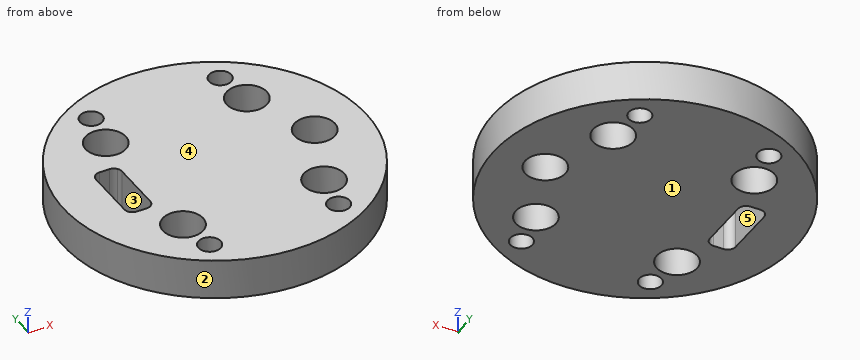
from build123d import *

# Parameters (mm, degrees)
SKETCH_1_R          = 37.5
EXTRUDE_1_DEPTH     = 10
SKETCH_2_R          = 5
CUT_EXTRUDE_1_DEPTH = 10
SKETCH_4_R          = 2.75
CUT_EXTRUDE_2_DEPTH = 10


with BuildPart() as part:
    # 草图1 → 凸台-拉伸1 (new body)
    with BuildSketch(Plane.XY):
        Circle(SKETCH_1_R)
        with BuildLine():
            ThreePointArc((-20.75113276, -17.528548354), (-17.528548354, -14.305963949), (-14.305963949, -17.528548354))
            ThreePointArc((-14.305963949, -17.528548354), (-17.528548354, -20.75113276), (-20.75113276, -17.528548354))
        make_face(mode=Mode.SUBTRACT)
        with BuildLine():
            ThreePointArc((14.305963949, -17.528548354), (17.528548354, -14.305963949), (20.75113276, -17.528548354))
            ThreePointArc((20.75113276, -17.528548354), (17.528548354, -20.75113276), (14.305963949, -17.528548354))
        make_face(mode=Mode.SUBTRACT)
        with BuildLine():
            Line((-24.045437487, 8.428297676), (-21.566526406, 8.428297676))
            ThreePointArc((-21.566526406, 8.428297676), (-20.68362959, 8.220920288), (-19.985383241, 7.642159365))
            ThreePointArc((-19.985383241, 7.642159365), (-19.686578169, 7.076512396), (-19.583397541, 6.445168811))
            Line((-19.583397541, 6.445168811), (-19.583397541, -6.445168811))
            ThreePointArc((-19.583397541, -6.445168811), (-20.164242538, -7.847452679), (-21.566526406, -8.428297676))
            Line((-21.566526406, -8.428297676), (-24.045437487, -8.428297676))
            ThreePointArc((-24.045437487, -8.428297676), (-25.447721356, -7.847452679), (-26.028566352, -6.445168811))
            Line((-26.028566352, -6.445168811), (-26.028566352, 6.445168811))
            ThreePointArc((-26.028566352, 6.445168811), (-25.447721356, 7.847452679), (-24.045437487, 8.428297676))
        make_face(mode=Mode.SUBTRACT)
        with BuildLine():
            ThreePointArc((-20.75113276, 17.528548354), (-17.528548354, 20.75113276), (-14.305963949, 17.528548354))
            ThreePointArc((-14.305963949, 17.528548354), (-17.528548354, 14.305963949), (-20.75113276, 17.528548354))
        make_face(mode=Mode.SUBTRACT)
        with BuildLine():
            ThreePointArc((14.305963949, 17.528548354), (17.528548354, 20.75113276), (20.75113276, 17.528548354))
            ThreePointArc((20.75113276, 17.528548354), (17.528548354, 14.305963949), (14.305963949, 17.528548354))
        make_face(mode=Mode.SUBTRACT)
        with BuildLine():
            ThreePointArc((21.814417514, 0), (24.789110812, 2.974693297), (27.763804109, 0))
            ThreePointArc((27.763804109, 0), (24.789110812, -2.974693297), (21.814417514, 0))
        make_face(mode=Mode.SUBTRACT)
    extrude(amount=EXTRUDE_1_DEPTH)

    # 草图2 → 切除-拉伸1 (cut)
    with BuildSketch(Plane.XY.offset(10)):
        with Locations((-17.528548354, 17.528548354)):
            Circle(SKETCH_2_R)
        with BuildLine():
            ThreePointArc((-20.75113276, 17.528548354), (-17.528548354, 14.305963949), (-14.305963949, 17.528548354))
            ThreePointArc((-14.305963949, 17.528548354), (-17.528548354, 20.75113276), (-20.75113276, 17.528548354))
        make_face(mode=Mode.SUBTRACT)
        with Locations((17.528548354, 17.528548354)):
            Circle(SKETCH_2_R)
        with BuildLine():
            ThreePointArc((20.75113276, 17.528548354), (17.528548354, 20.75113276), (14.305963949, 17.528548354))
            ThreePointArc((14.305963949, 17.528548354), (17.528548354, 14.305963949), (20.75113276, 17.528548354))
        make_face(mode=Mode.SUBTRACT)
        with Locations((-17.528548354, -17.528548354)):
            Circle(SKETCH_2_R)
        with BuildLine():
            ThreePointArc((-20.75113276, -17.528548354), (-17.528548354, -20.75113276), (-14.305963949, -17.528548354))
            ThreePointArc((-14.305963949, -17.528548354), (-17.528548354, -14.305963949), (-20.75113276, -17.528548354))
        make_face(mode=Mode.SUBTRACT)
        with Locations((17.528548354, -17.528548354)):
            Circle(SKETCH_2_R)
        with BuildLine():
            ThreePointArc((14.305963949, -17.528548354), (17.528548354, -20.75113276), (20.75113276, -17.528548354))
            ThreePointArc((20.75113276, -17.528548354), (17.528548354, -14.305963949), (14.305963949, -17.528548354))
        make_face(mode=Mode.SUBTRACT)
        with Locations((24.789110812, 0)):
            Circle(SKETCH_2_R)
        with BuildLine():
            ThreePointArc((21.814417514, 0), (24.789110812, -2.974693297), (27.763804109, 0))
            ThreePointArc((27.763804109, 0), (24.789110812, 2.974693297), (21.814417514, 0))
        make_face(mode=Mode.SUBTRACT)
    extrude(amount=-CUT_EXTRUDE_1_DEPTH, mode=Mode.SUBTRACT)

    # 草图4 → 切除-拉伸2 (cut)
    with BuildSketch(Plane.XY.offset(10)):
        with Locations((-16.071064876, -26.957760919)):
            Circle(SKETCH_4_R)
        with Locations((15.928824109, -27.042051743)):
            Circle(SKETCH_4_R)
        with Locations((16.071064876, 26.957760919)):
            Circle(SKETCH_4_R)
        with Locations((-15.928824109, 27.042051743)):
            Circle(SKETCH_4_R)
    extrude(amount=-CUT_EXTRUDE_2_DEPTH, mode=Mode.SUBTRACT)


solid = part.part
Design review of the part built by this model. Coordinates are the model's own, in mm. Face numbers are marked on the shaded views. A direction names the side the tool comes from. Round coordinates to 2 decimals unless told otherwise and drop trailing zeros. Write each loop counter-clockwise with the first axis right and the second up, starting at its lowest first coordinate (ties: lowest second). Pieces come first, ordered by that corner, then holes. Notation, with made-up numbers: (-24.75, -10.75) -> (-15.75, -10.75) arc R34 ccw to (-15.75, 23.25) -> close; hole circle Ø3 at (53, 80.5). An arc over 180 degrees is marked (long way). One line per item, written item: value. Start each with the question number.
Q1. To check wall thickness, follow probe 1 along X at (y, z) = (-16, 2); probe 2 along X at (y, z) = (-4, 4.5); probe 3 along Y at (x, z) = (15, 3.25). State the ranges of each line that lie inside material, in increasing order.
Q2. Add section C-C (z = 7.5). State how many separate pieces and enclosed holes the cut face has, then the cut area to 3 significant figures.
Q3. Add section D-D (y = -28). Give the boundary of the cut face in (x, z), then the cut area to 3 significant figures.
Q4. Tool access review of the marked faces 4 and 5: name each direction out of +Z, -Z, +X, -X, +Y, -Y from which nothing blocks a thin tool from reaching the whole face with its end or side.
Q5. Add section B-B (x = 28). Give the boundary of the cut face in (y, z).
Q6. Add section A-A (y = 0). Give the boundary of the cut face in (x, z), then the cut area to 3 significant figures.
Q7. The part is to be moulded in two halves that separate along Y. For the marked faces 1, 2 and 3, say which applies: pulls with the +Y half, pulls with the -Y half, needs draft (parallel to the pull), parting line crosses it, or undercut.
Q8. Insertion check: P1, Ø13, axis at x = 24.79, y = 0, coming from the -Z side; P2, Ø4, axis at y = 3, z = 3, coming from the -X side; P3, Ø0.7, axis at x = -22.5, z = 7.5, coming from the +Y side; P4, Ø4, axis at y = 22, z = 4, coming from the -X side. Each pin has a flat end and moves straight along its axis. Give the tip position at first contact, or say it passes through.
Response:
1. probe 1: x = -33.92 to -22.29, -12.77 to 12.77, 22.29 to 33.92
1. probe 2: x = -37.29 to -26.03, -19.58 to 21.79, 27.79 to 37.29
1. probe 3: y = -34.37 to -29.63, -24.45 to -21.84, -13.22 to 13.22, 21.84 to 24.42, 29.49 to 34.37
2. separate pieces: 1
2. enclosed holes: 10
2. area: 3,820 mm^2
3. outline: (-24.94, 0) -> (-18.62, 0) -> (-18.62, 10) -> (-24.94, 10) -> close; (-13.53, 0) -> (13.35, 0) -> (13.35, 10) -> (-13.53, 10) -> close; (18.51, 0) -> (24.94, 0) -> (24.94, 10) -> (18.51, 10) -> close
3. area: 396 mm^2
4. face 4: +Z, +X, -X, +Y, -Y
4. face 5: +Z, -Z
5. outline: (-24.94, 0) -> (-3.83, 0) -> (-3.83, 10) -> (-24.94, 10) -> close; (3.83, 0) -> (24.94, 0) -> (24.94, 10) -> (3.83, 10) -> close
6. outline: (-37.5, 0) -> (-26.03, 0) -> (-26.03, 10) -> (-37.5, 10) -> close; (-19.58, 0) -> (19.79, 0) -> (19.79, 10) -> (-19.58, 10) -> close; (29.79, 0) -> (37.5, 0) -> (37.5, 10) -> (29.79, 10) -> close
6. area: 586 mm^2
7. face 1: needs draft
7. face 2: parting line crosses it
7. face 3: undercut
8. P1: stops at z = 0
8. P2: stops at x = -37.49
8. P3: stops at y = 30.26
8. P4: stops at x = -31.72
